```python
from build123d import *

# Parameters (mm, degrees)
SKETCH1_W                                         = 100
SKETCH1_H                                         = 100
BOSS_EXTRUDE1_DEPTH                               = 20
CSK_FOR_1_FLAT_HEAD_MACHINE_SCREW_100_D           = 2.0574
CSK_FOR_1_FLAT_HEAD_MACHINE_SCREW_100_CSINK_D     = 3.7084
CSK_FOR_1_FLAT_HEAD_MACHINE_SCREW_100_CSINK_ANGLE = 100
F_1_0_228_DIAMETER_HOLE1_D                        = 5.7912


with BuildPart() as part:
    # Sketch1 → Boss-Extrude1 (new body)
    with BuildSketch(Plane(origin=(0, 0, 0), x_dir=(1, 0, 0), z_dir=(0, 1, 0))):
        with Locations((21.428571429, -2.857142857)):
            Rectangle(SKETCH1_W, SKETCH1_H)
    extrude(amount=BOSS_EXTRUDE1_DEPTH)

    # CSK for #1 Flat Head Machine Screw (100)1 (through all)
    with Locations(Plane(origin=(21.428571429, 0, -13.80952381), x_dir=(0, 0, -1), z_dir=(0, -1, 0))):
        with Locations((0, 0), (-33.333333334, 0)):
            CounterSinkHole(CSK_FOR_1_FLAT_HEAD_MACHINE_SCREW_100_D / 2, CSK_FOR_1_FLAT_HEAD_MACHINE_SCREW_100_CSINK_D / 2, counter_sink_angle=CSK_FOR_1_FLAT_HEAD_MACHINE_SCREW_100_CSINK_ANGLE)

    # #1 (0.228) Diameter Hole1 (through all)
    with Locations(Plane(origin=(-23.530488072, 20, 47.857142857), x_dir=(0, 0, 1), z_dir=(0, 1, 0))):
        with Locations((0, 0), (0, 89.959059501), (-90, 89.959059501), (-90, -0.040940499)):
            Hole(F_1_0_228_DIAMETER_HOLE1_D / 2)


solid = part.part
```
Geometry check sheet. Reference: the model listing, model coordinates, mm. Give positions to 0.01 mm unless a question says otherwise; leave off trailing zeros.
1. Release check for a two-part mould opening along Z. For faces 1 (the face through (68.87, 9.86, 46.3)), 2 (the face through (21, 10, -47.143)), 3 (the face through (21, 20, 2)) record: pulls with the +Z half, pulls with the -Z half, needs draft (parallel to the pull), parting line crosses it, or undercut.
2. Gauge pin test, flat end, axial feed: pin 1 Ø3.5 at (x, z) = (66.43, -42.14) entering from -Y. Record the tip position at first contact, or that the pin passes through.
3. Thickness scan on L1, parallel to X at y = 11.75, z = 19.5; L2, parallel to X at y = 2.25, z = 19. Record the ranges inside material, lowest first.
Values follow:
1. face 1: undercut
1. face 2: pulls with the -Z half
1. face 3: needs draft
2. pin 1: passes through
3. L1: x = -28.57 to 20.4, 22.46 to 71.43
3. L2: x = -28.57 to 20.54, 22.31 to 71.43
